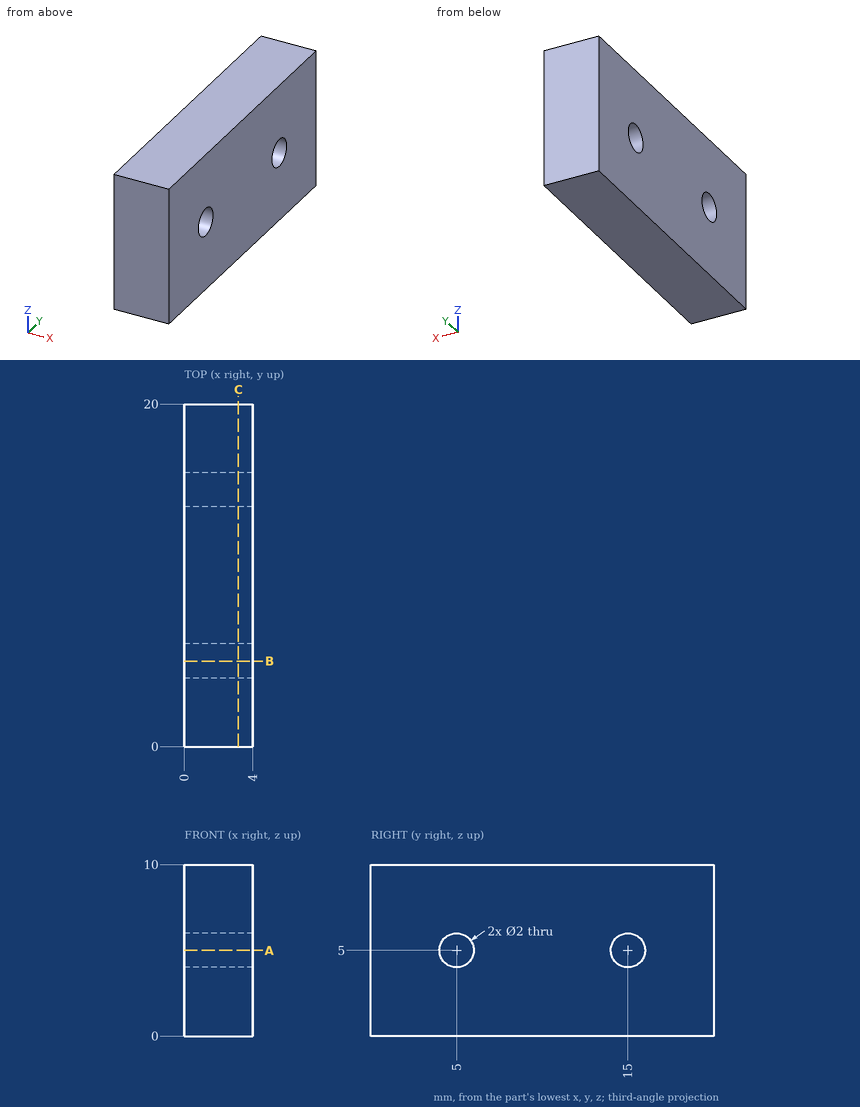
Could you check a few things on this drawing? It's one solid part, dimensions in mm from its lowest x, y, z. Round coordinates to 2 decimals unless told otherwise and drop trailing zeros. Order: outer loops, then holes, each group sorted by start corner. A loop starts at its lowest first (then second) coordinate and runs counter-clockwise, first axis right, second up. Notation, with made-up numbers: M 44.5,27 L 95.5,27 A21 cw 95.5,58 Z; hole C 87.5,75.25 d5. An arc over 180 degrees is marked long. One line per item, written item: value.
(1) Imagine slicing it at C-C (x = 3.15). Write out the boundary of the cut face in (y, z).
Ans:
outline: M 0,0 L 20,0 L 20,10 L 0,10 Z; hole C 5,5 d2; hole C 15,5 d2
(2) I need wall thicknesses on line 1 along Y through (x, z) = (2.75, 5); line 2 along Z through (x, y) = (2.55, 5); line 3 along Y through (x, z) = (3.15, 5.75). Which ranges of each line are inside material? Lowest first, please. Write a range as from..to.
Ans:
line 1: y = 0..4, 6..14, 16..20
line 2: z = 0..4, 6..10
line 3: y = 0..4.34, 5.66..14.34, 15.66..20
(3) Imagine slicing it at A-A (z = 5). Write out the boundary of the cut face in (x, y).
Ans:
outline: M 0,0 L 4,0 L 4,4 L 0,4 Z; M 0,6 L 4,6 L 4,14 L 0,14 Z; M 0,16 L 4,16 L 4,20 L 0,20 Z
(4) Imagine slicing it at B-B (y = 5). Write out the boundary of the cut face in (x, z).
Ans:
outline: M 0,0 L 4,0 L 4,4 L 0,4 Z; M 0,6 L 4,6 L 4,10 L 0,10 Z
(5) I'm going to push a flat-ended pin straight in: P1, Ø1.8, axis at y = 5, z = 5, coming from the -X side. Where does the tip first touch, or does it pass through?
Ans:
P1: passes through
